The listing builds one solid part. Answer for the finished solid, in the listing's coordinates (mm). A direction names the side the tool comes from. Coordinates: 2 decimals unless noted, no trailing zeros. Write each loop counter-clockwise with the first axis right and the second up, starting at its lowest first coordinate (ties: lowest second). Pieces come first, ordered by that corner, then holes.
from build123d import *

# Parameters (mm, degrees)
SKETCH1_R            = 1.75
BOSS_EXTRUDE1_DEPTH  = 10
CUT_EXTRUDE1_DEPTH   = 6
BOSS_EXTRUDE2_DEPTH  = 10
BOSS_EXTRUDE3_DEPTH  = 15.1
M3_CLEARANCE_HOLE1_D = 3.4
M3_CLEARANCE_HOLE2_D = 3.4


with BuildPart() as part:
    # Sketch1 → Boss-Extrude1 (new body)
    with BuildSketch(Plane.XY):
        with BuildLine():
            Line((-7.6, 10), (10.134969828, 10))
            ThreePointArc((10.134969828, 10), (11.498966548, 9.462707403), (12.130097928, 8.139512947))
            Line((12.130097928, 8.139512947), (12.279025895, 6.009743799))
            Line((12.279025895, 6.009743799), (122.011071424, 13.682955911))
            Line((122.011071424, 13.682955911), (122.011071424, 15.827693331))
            ThreePointArc((122.011071424, 15.827693331), (122.54836402, 17.191690051), (123.871558476, 17.822821431))
            Line((123.871558476, 17.822821431), (127.996455725, 18.111262346))
            ThreePointArc((127.996455725, 18.111262346), (129.448086731, 17.625553406), (130.131096773, 16.255647193))
            Line((130.131096773, 16.255647193), (130.513028814, 10.79376454))
            ThreePointArc((130.513028814, 10.79376454), (129.45752894, 7.356802052), (126.3687377, 5.516649939))
            Line((126.3687377, 5.516649939), (12, -14.058605554))
            Line((12, -14.058605554), (12, -21))
            ThreePointArc((12, -21), (10.535533906, -24.535533906), (7, -26))
            Line((7, -26), (-7.6, -26))
            ThreePointArc((-7.6, -26), (-11.135533906, -24.535533906), (-12.6, -21))
            Line((-12.6, -21), (-12.6, 5))
            ThreePointArc((-12.6, 5), (-11.135533906, 8.535533906), (-7.6, 10))
        make_face()
        Circle(SKETCH1_R, mode=Mode.SUBTRACT)
        with Locations((0, -18)):
            Circle(SKETCH1_R, mode=Mode.SUBTRACT)
    extrude(amount=BOSS_EXTRUDE1_DEPTH)

    # Sketch2 → Cut-Extrude1 (cut)
    with BuildSketch(Plane.XY.offset(10)):
        with BuildLine():
            Line((12, -5.257633034), (12, -1.749595529))
            ThreePointArc((12, -1.749595529), (13.074585194, 0.978397911), (15.720974105, 2.240660672))
            Line((15.720974105, 2.240660672), (100.359457674, 8.159159996))
            ThreePointArc((100.359457674, 8.159159996), (101.953365437, 6.84188311), (100.717151126, 5.18431425))
            Line((100.717151126, 5.18431425), (16.67482331, -9.20029882))
            ThreePointArc((16.67482331, -9.20029882), (13.421172092, -8.31535222), (12, -5.257633034))
        make_face()
    extrude(amount=-CUT_EXTRUDE1_DEPTH, mode=Mode.SUBTRACT)

    # Sketch4 → Boss-Extrude2 (add)
    with BuildSketch(Plane.XY.offset(10)):
        Polygon((12, -18.990256201), (48, -7.896876292), (12, -14.058605554), align=None)
    extrude(amount=-BOSS_EXTRUDE2_DEPTH)

    # Sketch5 → Boss-Extrude3 (add)
    with BuildSketch(Plane.XY.offset(10)):
        with BuildLine():
            Line((-7.6, 7.5), (-7.6, -26))
            ThreePointArc((-7.6, -26), (-11.135533906, -24.535533906), (-12.6, -21))
            Line((-12.6, -21), (-12.6, 5))
            ThreePointArc((-12.6, 5), (-11.135533906, 8.535533906), (-7.6, 10))
            Line((-7.6, 10), (10.134969828, 10))
            ThreePointArc((10.134969828, 10), (11.498966548, 9.462707403), (12.130097928, 8.139512947))
            Line((12.130097928, 8.139512947), (12.279025895, 6.009743799))
            Line((12.279025895, 6.009743799), (7.5, 6.009743799))
            Line((7.5, 6.009743799), (7.5, 7.5))
            Line((7.5, 7.5), (-7.6, 7.5))
        make_face()
    extrude(amount=BOSS_EXTRUDE3_DEPTH)

    # M3 Clearance Hole1 (through all)
    with Locations(Plane(origin=(-7.6, 0, 0), x_dir=(0, 0, -1), z_dir=(1, 0, 0))):
        with Locations((-17.6, -18), (-17.6, 0)):
            Hole(M3_CLEARANCE_HOLE1_D / 2)

    # M3 Clearance Hole2 (through all)
    with Locations(Plane(origin=(0, 10, 0), x_dir=(1, 0, 0), z_dir=(0, 1, 0))):
        with Locations((0, -17.6)):
            Hole(M3_CLEARANCE_HOLE2_D / 2)


solid = part.part
Q1. Find the intervals of material crossed by probe 1 along Y at (x, z) = (-10.35, 17.6); probe 2 along Z at (x, y) = (15, -17); probe 3 along Z at (x, y) = (0, 8.4), in increasing order.
Answers below:
probe 1: y = -25.18 to -19.7, -16.3 to -1.7, 1.7 to 9.18
probe 2: z = 0 to 10
probe 3: z = 0 to 15.9, 19.3 to 25.1
Q2. Which of the six approach directions +Z, -Z, +X, -X, +Y, -Y give full straight-line access (tool end or side, diameter ignored) to faces 4 (the face through (13.05, 0.95, 7.04)), 5 (the face through (1, 10, 12)), 6 (the face through (10, 6.01, 17)), 7 (the face through (-0.228, -16.265, 4.93))?
Answers below:
face 4: +Z
face 5: +Z, -Z, -X, +Y
face 6: +Z, +X, -Y
face 7: +Z, -Z
Q3. The part is cut by section A-A, the plane z = 17.6. Write down the section's boundary in (x, y).
Answers below:
outline: (-12.6, -21) arc R5 ccw to (-7.6, -26) - (-7.6, -19.7) - (-12.6, -19.7) - close; (-12.6, -16.3) - (-7.6, -16.3) - (-7.6, -1.7) - (-12.6, -1.7) - close; (-12.6, 1.7) - (-7.6, 1.7) - (-7.6, 7.5) - (-1.7, 7.5) - (-1.7, 10) - (-7.6, 10) arc R5 ccw to (-12.6, 5) - close; (1.7, 7.5) - (7.5, 7.5) - (7.5, 6.01) - (12.28, 6.01) - (12.13, 8.14) arc R2 ccw to (10.13, 10) - (1.7, 10) - close
Q4. The part is cut by section C-C, the plane y = 0. Write down the section's boundary in (x, z).
Answers below:
outline: (-12.6, 0) - (-1.75, 0) - (-1.75, 10) - (-7.6, 10) - (-7.6, 15.9) - (-12.6, 15.9) - close; (-12.6, 19.3) - (-7.6, 19.3) - (-7.6, 25.1) - (-12.6, 25.1) - close; (1.75, 0) - (94.14, 0) - (94.14, 10) - (70.43, 10) - (70.43, 4) - (12.4, 4) - (12.4, 10) - (1.75, 10) - close
Q5. Determine the mould class of faces 1 (the face through (130.32, 13.56, 4.93)), 2 (the face through (48, 0, 4)), 3 (the face through (-12.6, -8, 12)) for opening direction X: released by +X, released by -X, zero draft, split by the parting line, or undercut.
Answers below:
face 1: released by +X
face 2: undercut
face 3: released by -X
Q6. The part is cut by section D-D, the plane x = 36. Write down the section's boundary in (y, z).
Answers below:
outline: (-11.59, 0) - (7.67, 0) - (7.67, 10) - (3.66, 10) - (3.66, 4) - (-5.89, 4) - (-5.89, 10) - (-11.59, 10) - close
Q7. Given pin 1 (0.7 mm diameter, centred on y = 7, z = 19, fed in from -X); pin 2 (3 mm diameter, centred on y = -18, z = 17.6, fed in from -X); pin 3 (1.5 mm diameter, centred on y = -14, z = 11, fed in from +X); pin 4 (14 mm diameter, centred on x = 0, z = 15.5, fed in from +Y), each flat-ended and moving along its own axis, determine where each tip first touches the part or whether it passes through.
Answers below:
pin 1: stops at x = -12.32
pin 2: passes through
pin 3: stops at x = -7.6
pin 4: stops at y = 10
Q8. The part is cut by section B-B, the plane x = 0. Write down the section's boundary in (y, z).
Answers below:
outline: (-26, 0) - (-19.75, 0) - (-19.75, 10) - (-26, 10) - close; (-16.25, 0) - (-1.75, 0) - (-1.75, 10) - (-16.25, 10) - close; (1.75, 0) - (10, 0) - (10, 15.9) - (7.5, 15.9) - (7.5, 10) - (1.75, 10) - close; (7.5, 19.3) - (10, 19.3) - (10, 25.1) - (7.5, 25.1) - close
